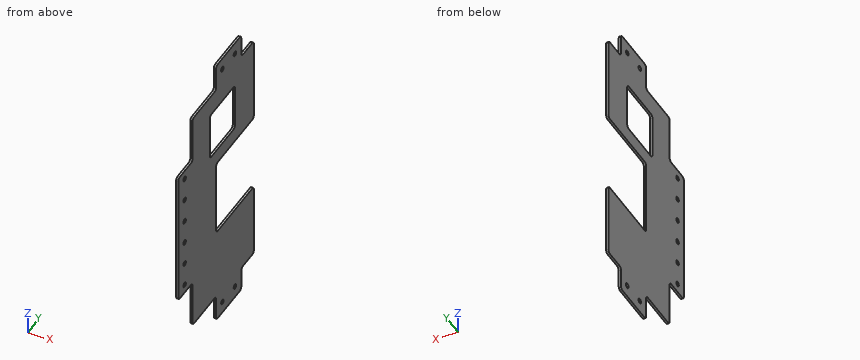
Autodesk Inventor part; units mm, degrees
ref_plane "YZ Plane" through (0, 0, 0) normal (1, 0, 0) x (0, 1, 0)
ref_plane "XZ Plane" through (0, 0, 0) normal (0, 1, 0) x (-1, 0, 0)
ref_plane "XY Plane" through (0, 0, 0) normal (0, 0, 1) x (1, 0, 0)
sketch "Sketch1" plane through (0, 0, 0) normal (1, 0, 0) x (0, 1, 0)
  line L0 (76.2, 152.4) -> (-76.2, 152.4)
  line L1 (-76.2, 152.4) -> (-76.2, -152.4)
  line L2 (-76.2, -152.4) -> (76.2, -152.4)
  line L3 (76.2, -152.4) -> (76.2, 152.4)
  line L4 (76.2, 152.4) -> (-76.2, -152.4) construction
  line L5 (-76.2, 152.4) -> (76.2, -152.4) construction
  line L6 (38.1, 101.6) -> (-12.7, 101.6)
  line L7 (-12.7, 101.6) -> (-12.7, 50.8)
  line L8 (-12.7, 50.8) -> (38.1, 50.8)
  line L9 (38.1, 50.8) -> (38.1, 101.6)
  line L10 (38.1, 101.6) -> (-12.7, 50.8) construction
  line L11 (-12.7, 101.6) -> (38.1, 50.8) construction
  line L12 (76.2, 34.925) -> (0, 34.925)
  line L13 (0, 34.925) -> (0, -47.625)
  line L14 (0, -47.625) -> (76.2, -47.625)
  line L15 (76.2, -47.625) -> (76.2, 34.925)
  line L16 (76.2, 34.925) -> (0, -47.625) construction
  line L17 (0, 34.925) -> (76.2, -47.625) construction
  point P0 (0, 0)
  point P1 (12.7, 76.2)
  point P2 (38.1, -6.35)
  point P3 (76.2, -6.35)
  point P4 (76.2, 0)
  point P5 (76.2, -47.625)
  point P6 (0, 44.45)
  point P7 (31.75, 44.45)
  point P8 (76.2, 34.925)
  dimension "d0" = 152.4
  dimension "d1" = 304.8
  dimension "d2" = 50.8
  dimension "d3" = 88.9
  dimension "d4" = 76.2
  dimension "d39" = 76.2
  dimension "d40" = 82.55
  dimension "d41" = 146.05
extrude "Extrusion1" add sketch "Sketch1" along normal blind 2.286 contours L3 L12 L13 L14 L2 L1 L0
fillet "Fillet1" radius 3.175 8 edges at (1.143, 38.1, 50.8) (1.143, 38.1, 101.6) (1.143, -12.7, 101.6) (1.143, -12.7, 50.8) (1.143, 76.2, 152.4) (1.143, 76.2, -152.4) (1.143, -76.2, -152.4) (1.143, -76.2, 152.4)
sketch "Sketch2" plane through (2.286, 0, 0) normal (1, 0, 0) x (0, 0, -1)
  arc A0 (-152.4, -73.025) -> (-149.225, -76.2) centre (-149.225, -73.025) ccw construction
  line L0 (-152.4, -73.025) -> (-152.4, 73.025) construction
  arc A1 (-149.225, 76.2) -> (-152.4, 73.025) centre (-149.225, 73.025) ccw construction
  line L1 (-149.225, 76.2) -> (-34.925, 76.2) construction
  arc A2 (152.4, 73.025) -> (149.225, 76.2) centre (149.225, 73.025) ccw construction
  line L2 (152.4, 73.025) -> (152.4, -73.025) construction
  arc A3 (149.225, -76.2) -> (152.4, -73.025) centre (149.225, -73.025) ccw construction
  line L3 (149.225, -76.2) -> (-149.225, -76.2) construction
  line L4 (-34.925, 76.2) -> (-34.925, 0)
  line L5 (-34.925, 0) -> (47.625, 0)
  line L6 (47.625, 0) -> (47.625, 76.2)
  line L7 (47.625, 76.2) -> (149.225, 76.2)
  arc A4 (-53.975, -12.7) -> (-50.8, -9.525) centre (-53.975, -9.525) ccw
  line L8 (-50.8, -9.525) -> (-50.8, 34.925)
  arc A5 (-50.8, 34.925) -> (-53.975, 38.1) centre (-53.975, 34.925) ccw
  line L9 (-53.975, 38.1) -> (-98.425, 38.1)
  arc A6 (-98.425, 38.1) -> (-101.6, 34.925) centre (-98.425, 34.925) ccw
  line L10 (-101.6, 34.925) -> (-101.6, -9.525)
  arc A7 (-101.6, -9.525) -> (-98.425, -12.7) centre (-98.425, -9.525) ccw
  line L11 (-98.425, -12.7) -> (-53.975, -12.7)
  point P0 (0, 0)
  point P1 (-139.7, -63.5)
  point P2 (139.7, -63.5)
  point P3 (-139.7, -38.1)
  point P4 (139.7, -38.1)
  point P5 (-139.7, -12.7)
  point P6 (139.7, -12.7)
  point P7 (-139.7, 12.7)
  point P8 (139.7, 12.7)
  point P9 (-139.7, 38.1)
  point P10 (139.7, 38.1)
  point P11 (-139.7, 63.5)
  point P12 (139.7, 63.5)
  point P13 (-114.3, -63.5)
  point P14 (-88.9, -63.5)
  point P15 (-63.5, -63.5)
  point P16 (-38.1, -63.5)
  point P17 (-12.7, -63.5)
  point P18 (12.7, -63.5)
  point P19 (38.1, -63.5)
  point P20 (63.5, -63.5)
  point P21 (88.9, -63.5)
  point P22 (114.3, -63.5)
  point P23 (139.7, -63.5)
  dimension "d8" = 12.7
  dimension "d9" = 12.7
  dimension "d10" = 12.7
  dimension "d13" = 25.4
  dimension "d34" = 25.4
hole "Hole1" at (2.286, -63.5, 139.7) at (2.286, -63.5, -139.7) at (2.286, -38.1, 139.7) at (2.286, -38.1, -139.7) at (2.286, -12.7, 139.7) at (2.286, -12.7, -139.7) at (2.286, 12.7, 139.7) at (2.286, 12.7, -139.7) at (2.286, 38.1, 139.7) at (2.286, 38.1, -139.7) at (2.286, 63.5, 139.7) at (2.286, 63.5, -139.7) at (2.286, -63.5, 88.9) at (2.286, -63.5, 63.5) at (2.286, -63.5, 38.1) at (2.286, -63.5, 12.7) at (2.286, -63.5, -12.7) at (2.286, -63.5, -38.1) at (2.286, -63.5, -63.5) at (2.286, -63.5, -88.9) direction (-1, 0, 0) diameter 5.1054 end through all
sketch "Sketch3" plane through (2.286, 0, 0) normal (1, 0, 0) x (0, 0, -1)
  line L0 (-123.825, 0) -> (-152.4, 0)
  line L1 (-152.4, 0) -> (-152.4, -76.2)
  line L2 (-152.4, -76.2) -> (-123.825, -76.2)
  line L3 (-123.825, -76.2) -> (-123.825, 0)
  line L4 (-123.825, 0) -> (-152.4, -76.2) construction
  line L5 (-152.4, 0) -> (-123.825, -76.2) construction
  circle A0 centre (-139.7, 63.5) radius 2.5527 construction
  circle A1 centre (-139.7, 38.1) radius 2.5527 construction
  circle A2 centre (-139.7, 12.7) radius 2.5527 construction
  circle A3 centre (-139.7, -12.7) radius 2.5527 construction
  circle A4 centre (-139.7, -38.1) radius 2.5527 construction
  circle A5 centre (-139.7, -63.5) radius 2.5527 construction
  circle A6 centre (139.7, -63.5) radius 2.5527 construction
  circle A7 centre (139.7, -38.1) radius 2.5527 construction
  circle A8 centre (139.7, -12.7) radius 2.5527 construction
  circle A9 centre (139.7, 12.7) radius 2.5527 construction
  circle A10 centre (139.7, 38.1) radius 2.5527 construction
  circle A11 centre (139.7, 63.5) radius 2.5527 construction
  arc A12 (-152.4, -73.025) -> (-149.225, -76.2) centre (-149.225, -73.025) ccw construction
  line L6 (-152.4, -73.025) -> (-152.4, 73.025) construction
  arc A13 (-149.225, 76.2) -> (-152.4, 73.025) centre (-149.225, 73.025) ccw construction
  line L7 (-149.225, 76.2) -> (-34.925, 76.2) construction
  arc A14 (152.4, 73.025) -> (149.225, 76.2) centre (149.225, 73.025) ccw construction
  line L8 (152.4, 73.025) -> (152.4, -73.025) construction
  arc A15 (149.225, -76.2) -> (152.4, -73.025) centre (149.225, -73.025) ccw construction
  line L9 (149.225, -76.2) -> (-149.225, -76.2) construction
  line L10 (-149.225, -76.2) -> (149.225, -76.2) construction
  line L11 (149.225, 76.2) -> (-149.225, 76.2) construction
  line L12 (0, 76.2) -> (0, -76.2) construction
  line L13 (-149.225, -76.2) -> (149.225, -76.2) construction
  line L14 (-152.4, -47.625) -> (-73.025, -47.625)
  line L15 (-73.025, -47.625) -> (-73.025, -76.2)
  line L16 (-73.025, -76.2) -> (-152.4, -76.2)
  line L17 (-152.4, -76.2) -> (-152.4, -47.625)
  line L18 (-152.4, -47.625) -> (-73.025, -76.2) construction
  line L19 (-73.025, -47.625) -> (-152.4, -76.2) construction
  line L20 (123.825, 0) -> (152.4, 0)
  line L21 (152.4, 0) -> (152.4, -76.2)
  line L22 (152.4, -76.2) -> (123.825, -76.2)
  line L23 (123.825, -76.2) -> (123.825, 0)
  line L24 (123.825, 0) -> (152.4, -76.2) construction
  line L25 (152.4, 0) -> (123.825, -76.2) construction
  circle A16 centre (139.7, -12.7) radius 2.5527 construction
  circle A17 centre (139.7, -38.1) radius 2.5527 construction
  circle A18 centre (139.7, -63.5) radius 2.5527 construction
  arc A19 (149.225, -76.2) -> (152.4, -73.025) centre (149.225, -73.025) ccw construction
  arc A20 (98.425, -25.4) -> (101.6, -22.225) centre (98.425, -22.225) ccw construction
  line L26 (152.4, -47.625) -> (73.025, -47.625)
  line L27 (73.025, -47.625) -> (73.025, -76.2)
  line L28 (73.025, -76.2) -> (152.4, -76.2)
  line L29 (152.4, -76.2) -> (152.4, -47.625)
  line L30 (152.4, -47.625) -> (73.025, -76.2) construction
  line L31 (73.025, -47.625) -> (152.4, -76.2) construction
  circle A21 centre (63.5, -63.5) radius 2.5527
  circle A22 centre (12.7, -63.5) radius 2.5527
  circle A23 centre (-38.1, -63.5) radius 2.5527
  circle A24 centre (-88.9, -63.5) radius 2.5527
  circle A25 centre (-63.5, -63.5) radius 2.5527
  circle A26 centre (-12.7, -63.5) radius 2.5527
  circle A27 centre (38.1, -63.5) radius 2.5527
  circle A28 centre (88.9, -63.5) radius 2.5527
  line L32 (-34.925, 76.2) -> (-34.925, 0)
  line L33 (-34.925, 0) -> (47.625, 0)
  line L34 (47.625, 0) -> (47.625, 76.2)
  line L35 (47.625, 76.2) -> (149.225, 76.2)
  arc A29 (-53.975, -12.7) -> (-50.8, -9.525) centre (-53.975, -9.525) ccw
  line L36 (-50.8, -9.525) -> (-50.8, 34.925)
  arc A30 (-50.8, 34.925) -> (-53.975, 38.1) centre (-53.975, 34.925) ccw
  line L37 (-53.975, 38.1) -> (-98.425, 38.1)
  arc A31 (-98.425, 38.1) -> (-101.6, 34.925) centre (-98.425, 34.925) ccw
  line L38 (-101.6, 34.925) -> (-101.6, -9.525)
  arc A32 (-101.6, -9.525) -> (-98.425, -12.7) centre (-98.425, -9.525) ccw
  line L39 (-98.425, -12.7) -> (-53.975, -12.7)
  line L40 (-127, 50.8) -> (-152.4, 50.8)
  line L41 (-152.4, 50.8) -> (-152.4, 76.2)
  line L42 (-152.4, 76.2) -> (-127, 76.2)
  line L43 (-127, 76.2) -> (-127, 50.8)
  circle A33 centre (139.7, 63.5) radius 2.5527 construction
  arc A34 (152.4, 73.025) -> (149.225, 76.2) centre (149.225, 73.025) ccw construction
  line L44 (127, 50.8) -> (152.4, 50.8)
  line L45 (152.4, 50.8) -> (152.4, 76.2)
  line L46 (152.4, 76.2) -> (127, 76.2)
  line L47 (127, 76.2) -> (127, 50.8)
  point P0 (0, 0)
  point P1 (-138.1125, -38.1)
  point P2 (-101.6, -22.225)
  point P3 (-98.425, -25.4)
  point P4 (-98.425, -22.225)
  point P5 (-112.7125, -61.9125)
  point P6 (138.1125, -38.1)
  point P7 (112.7125, -61.9125)
  point P8 (123.825, -47.625)
  point P9 (-123.825, -47.625)
  dimension "d25" = 28.575
  dimension "d26" = 76.2
  dimension "d27" = 28.575
  dimension "d28" = 79.375
  dimension "d42" = 25.4
extrude "Extrusion2" cut sketch "Sketch3" against normal through all contours L3 L14 L1 L0 | L14 L15 L16 L3 | L3 L2 L1 L14 | L20 L21 L26 L23 | L26 L21 L22 L23 | L23 L28 L27 L26 | A24 | A28 | L35 L46 L45 L44 L47 | L40 L41 L42 L43
fillet "Fillet2" radius 3.175 20 edges at (1.143, 0, 152.4) (1.143, 0, 123.825) (1.143, -47.625, 123.825) (1.143, -47.625, 73.025) (1.143, -76.2, 73.025) (1.143, -76.2, -73.025) (1.143, -47.625, -73.025) (1.143, -47.625, -123.825) (1.143, 0, -123.825) (1.143, 0, -152.4) (1.143, 0, 34.925) (1.143, 0, -47.625) (1.143, 76.2, -47.625) (1.143, 76.2, 34.925) (1.143, 50.8, 127) (1.143, 76.2, 127) (1.143, 50.8, 152.4) (1.143, 76.2, -127) (1.143, 50.8, -127) (1.143, 50.8, -152.4)
properties part number "DB1-025" material "Polycarbonate, Smoke"
Source: CAD feature listing. Evaluate the final solid. Frame: model axes, mm. Give positions to 0.01 mm unless a question says otherwise; leave off trailing zeros. Write each loop counter-clockwise with the first axis right and the second up, starting at its lowest first coordinate (ties: lowest second). Pieces come first, ordered by that corner, then holes. Notation, with made-up numbers: (14.5, 28) - (71.5, 28) arc R21 ccw to (71.5, 53) - close; hole circle Ø5 at (-39, -15). An arc over 180 degrees is marked (long way). One line per item, written item: value. Start each with the question number.
Q1. Material intervals for probe 1 along Y at (x, z) = (1.35, -139.7); probe 2 along Y at (x, z) = (1.2, -12.7); probe 3 along Z at (x, y) = (2, 67) (3 decimals), sorted ascending. Write a range as from..to.
Q2. First-contact query: pin 1 Ø0.7 at (x, z) = (1.5, 136) entering from -Y; pin 2 Ø0.7 at (x, y) = (0.5, 64.5) entering from +Z. Flat tips, straight axial feed; report the tip coordinate or a pass-through.
Q3. Section query D-D, the plane y = -27. Return the cut outline in (x, z) (3 decimals).
Q4. Section query A-A, the plane y = 26. Return the cut outline in (x, z) (3 decimals), then the cut area to 3 significant figures.
Q5. Section query C-C, the plane z = 114. Return the cut outline in (x, y) (3 decimals), then the cut area to 3 significant figures.
Q6. Section query B-B, the plane x = 1.15. Count the separate pieces of the cut face and the enclosed holes in it, then the cut area to 3 significant figures.
Answer:
1. probe 1: y = 0..10.15, 15.25..35.55, 40.65..50.8
1. probe 2: y = -76.2..-66.05, -60.95..0
1. probe 3: z = -127..-47.625, 34.925..127
2. pin 1: stops at y = 0
2. pin 2: stops at z = 127
3. outline: (0, -123.825) - (2.286, -123.825) - (2.286, 123.825) - (0, 123.825) - close
4. outline: (0, -152.4) - (2.286, -152.4) - (2.286, -47.625) - (0, -47.625) - close; (0, 34.925) - (2.286, 34.925) - (2.286, 50.8) - (0, 50.8) - close; (0, 101.6) - (2.286, 101.6) - (2.286, 152.4) - (0, 152.4) - close
4. area: 392 mm2
5. outline: (0, -47.625) - (2.286, -47.625) - (2.286, 76.2) - (0, 76.2) - close
5. area: 283 mm2
6. separate pieces: 1
6. enclosed holes: 11
6. area: 28,800 mm2
